Verification items for the finished model (mm, model axes). Face numbers are marked on the shaded views. A direction names the side the tool comes from. Give positions to 0.01 mm unless a question says otherwise; leave off trailing zeros. Loops run counter-clockwise (first coordinate to the right, second up) from the corner with the lowest first, then second, coordinate; pieces in that order, holes last. Notation, with made-up numbers: (29, 86.25) -> (75, 86.25) arc R26 cw to (75, 106.25) -> close; hole circle Ø4 at (-5, -1). An arc over 180 degrees is marked (long way). Answer in a Markdown table with one row per item. Add a question column.
Q1. Release check for a two-part mould opening along X. For the marked faces 1, 2, 3 and 4 record: pulls with the +X half, pulls with the -X half, needs draft (parallel to the pull), parting line crosses it, or undercut.
Q2. Section check A-A on z = 11.75. Enter the section's corners in (x, y).
Q3. Section check B-B on x = -11.75. Enter the section's corners in (y, z), and give its area (4 significant figures).
Q4. Gauge pin test, flat ends, axial feed: P1, Ø16, axis at x = 4, z = 3, coming from the +Y side; P2, Ø12, axis at x = 0, z = 0, coming from the +Y side. Record the tip position at first contact, or that the pin passes through.
Q5. Section check D-D on z = -11.75. Enter the section's corners in (x, y).
Q6. Set-up check for the marked faces 5 and 6: record each of +Z, -Z, +X, -X, +Y, -Y from which the full face is reachable in a straight line by a thin tool's end or side.
Q7. Material ranges on probe 1 along X at (y, z) = (5.75, -11.75); probe 2 along Z at (x, y) = (13, 9.5); probe 3 along Y at (x, z) = (0, 12.1), recorded low to high.
Q8. Section check C-C on y = 5. Enter the section's corners in (x, z), and give its area (3 significant figures).
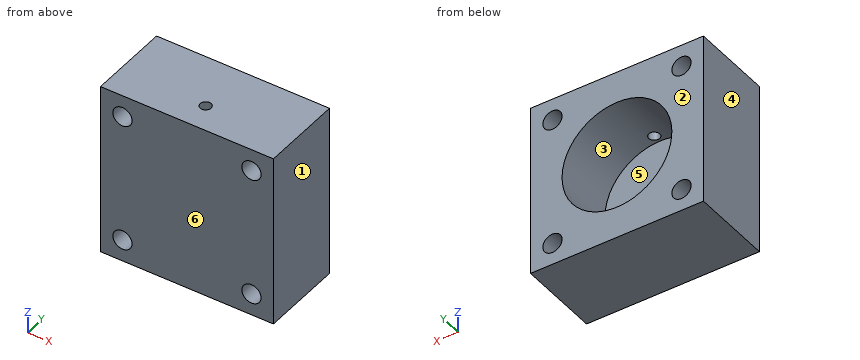
```python
from build123d import *

# Parameters (mm, degrees)
CROQUIS1_W                 = 31.5
CROQUIS1_H                 = 31.5
SALIENTE_EXTRUIR1_DEPTH    = 15
CROQUIS3_R                 = 10
CORTAR_EXTRUIR1_DEPTH      = 11.5
CROQUIS6_R                 = 1.75
CORTAR_EXTRUIR2_DEPTH      = 27.853770685
CORTAR_EXTRUIR3_REACH      = 40.279
CORTAR_EXTRUIR3_END_RADIUS = 10
CROQUIS7_R                 = 1


with BuildPart() as part:
    # Croquis1 → Saliente-Extruir1 (new body)
    with BuildSketch(Plane(origin=(0, 0, 0), x_dir=(1, 0, 0), z_dir=(0, 1, 0))):
        Rectangle(CROQUIS1_W, CROQUIS1_H)
    extrude(amount=SALIENTE_EXTRUIR1_DEPTH)

    # Croquis3 → Cortar-Extruir1 (cut)
    with BuildSketch(Plane(origin=(0, 15, 0), x_dir=(1, 0, 0), z_dir=(0, 1, 0))):
        with Locations(Location((0, 0, 0), (0, 0, 270))):
            Circle(CROQUIS3_R)
    extrude(amount=-CORTAR_EXTRUIR1_DEPTH, mode=Mode.SUBTRACT)

    # Croquis6 → Cortar-Extruir2 (cut, through all)
    with BuildSketch(Plane(origin=(0, 15, 0), x_dir=(1, 0, 0), z_dir=(0, 1, 0))):
        with Locations(Location((-11.75, -11.75, 0), (0, 0, 270))):
            Circle(CROQUIS6_R)
        with Locations(Location((11.75, -11.75, 0), (0, 0, 90))):
            Circle(CROQUIS6_R)
        with Locations(Location((11.75, 11.75, 0), (0, 0, 270))):
            Circle(CROQUIS6_R)
        with Locations(Location((-11.75, 11.75, 0), (0, 0, 90))):
            Circle(CROQUIS6_R)
    extrude(amount=-CORTAR_EXTRUIR2_DEPTH, mode=Mode.SUBTRACT)

    # Cortar-Extruir3: up to this cylinder (the profile starts outside it)
    cortar_extruir3_end = Plane(origin=(0, 5, 0), z_dir=(0, 1, 0)) * Cylinder(CORTAR_EXTRUIR3_END_RADIUS, 101.558, mode=Mode.PRIVATE)
    # Croquis7 → Cortar-Extruir3 (cut, up to the surface)
    with BuildSketch(Plane.XY.offset(15.75), mode=Mode.PRIVATE) as cortar_extruir3_sk1:
        with Locations((0, 5)):
            Circle(CROQUIS7_R)
    cortar_extruir3_tool1 = extrude(cortar_extruir3_sk1.sketch, amount=-CORTAR_EXTRUIR3_REACH, mode=Mode.PRIVATE) - cortar_extruir3_end
    add(cortar_extruir3_tool1.solids().sort_by_distance((0, 5, 15.75))[0], mode=Mode.SUBTRACT)


solid = part.part
```
Taken from the geometry:
| question | item | result |
|---|---|---|
| 1 | face 1 | pulls with the +X half |
| 1 | face 2 | needs draft |
| 1 | face 3 | undercut |
| 1 | face 4 | pulls with the -X half |
| 2 | outline | (-15.75, 0) -> (-13.5, 0) -> (-13.5, 15) -> (-15.75, 15) -> close; (-10, 0) -> (10, 0) -> (10, 15) -> (-10, 15) -> close; (13.5, 0) -> (15.75, 0) -> (15.75, 15) -> (13.5, 15) -> close; hole circle Ø2 at (0, 5) |
| 3 | outline | (0, -15.75) -> (15, -15.75) -> (15, -13.5) -> (0, -13.5) -> close; (0, -10) -> (15, -10) -> (15, 10) -> (0, 10) -> close; (0, 13.5) -> (15, 13.5) -> (15, 15.75) -> (0, 15.75) -> close |
| 3 | area | 367.5 mm² |
| 4 | P1 | stops at y = 15 |
| 4 | P2 | stops at y = 3.5 |
| 5 | outline | (-15.75, 0) -> (-13.5, 0) -> (-13.5, 15) -> (-15.75, 15) -> close; (-10, 0) -> (10, 0) -> (10, 15) -> (-10, 15) -> close; (13.5, 0) -> (15.75, 0) -> (15.75, 15) -> (13.5, 15) -> close |
| 6 | face 5 | +Y |
| 6 | face 6 | +Z, -Z, +X, -X, -Y |
| 7 | probe 1 | x = -15.75 to -13.5, -10 to 10, 13.5 to 15.75 |
| 7 | probe 2 | z = -15.75 to -12.97, -10.53 to 10.53, 12.97 to 15.75 |
| 7 | probe 3 | y = 0 to 4, 6 to 15 |
| 8 | outline | (-15.75, -15.75) -> (15.75, -15.75) -> (15.75, 15.75) -> (1, 15.75) -> (1, 9.95) arc R10 cw (long way) to (-1, 9.95) -> (-1, 15.75) -> (-15.75, 15.75) -> close; hole circle Ø3.5 at (-11.75, -11.75); hole circle Ø3.5 at (-11.75, 11.75); hole circle Ø3.5 at (11.75, -11.75); hole circle Ø3.5 at (11.75, 11.75) |
| 8 | area | 628 mm² |
